Geometry check sheet. Reference: drawing and pictorial views, mm from the part's lowest x, y, z. A direction names the side the tool comes from. Round coordinates to 2 decimals unless told otherwise and drop trailing zeros. Write each loop counter-clockwise with the first axis right and the second up, starting at its lowest first coordinate (ties: lowest second). Pieces come first, ordered by that corner, then holes. Notation, with made-up numbers: (-38, 36) -> (8, 36) arc R24 ccw to (8, 59) -> close; hole circle Ø9 at (-2, 83.5). An arc over 180 degrees is marked (long way). Write item = value, one per line.
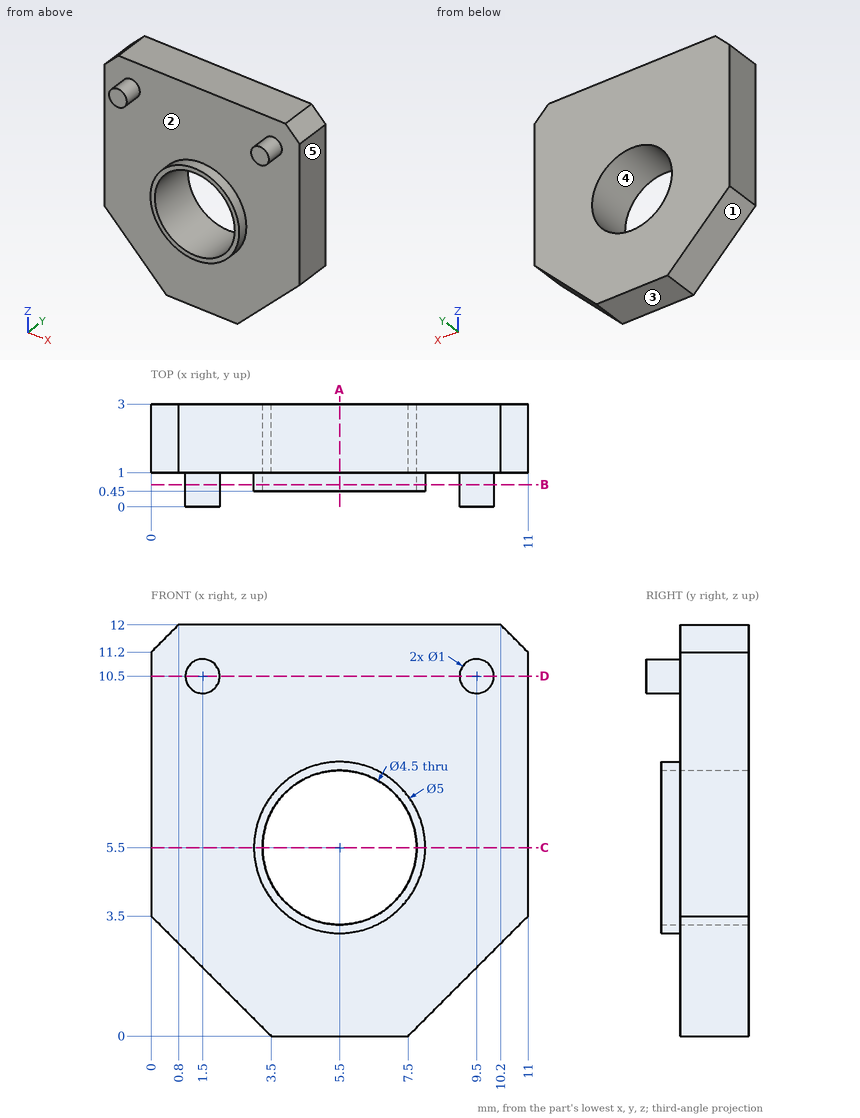
(1) Access from +Z, -Z, +X, -X, +Y, -Y to the whole of each face (thin tool, end or side, straight path). Record for the marked faces 1 and 2.
Worked answers:
face_1 = -Z, -X, +Y, -Y
face_2 = -Y
(2) Sectioned sample at A-A on x = 5.5. Enter the section's corners in (y, z), then the cut area to 3 significant figures.
Worked answers:
outline = (0.45, 3) -> (1, 3) -> (1, 0) -> (3, 0) -> (3, 3.25) -> (0.45, 3.25) -> close; (0.45, 7.75) -> (3, 7.75) -> (3, 12) -> (1, 12) -> (1, 8) -> (0.45, 8) -> close
area = 15.3 mm²
(3) Sectioned sample at D-D on z = 10.5. Enter the section's corners in (x, y).
Worked answers:
outline = (0, 1) -> (1, 1) -> (1, 0) -> (2, 0) -> (2, 1) -> (9, 1) -> (9, 0) -> (10, 0) -> (10, 1) -> (11, 1) -> (11, 3) -> (0, 3) -> close
(4) Material ranges on L1, parallel to Z at x = 5.5, y = 1.2; L2, parallel to X at y = 1.35, z = 5.5; L3, parallel to Z at x = 9.5, y = 2.55, recorded low to high. Write a range as [from, to].
Worked answers:
L1 = [0, 3.25], [7.75, 12]
L2 = [0, 3.25], [7.75, 11]
L3 = [2, 12]
(5) Release check for a two-part mould opening along X. For the marked faces 3, 4 and 5 record: pulls with the +X half, pulls with the -X half, needs draft (parallel to the pull), parting line crosses it, or undercut.
Worked answers:
face_3 = needs draft
face_4 = undercut
face_5 = pulls with the +X half
(6) Sectioned sample at B-B on y = 0.65. Enter the section's corners in (x, z), then the cut area to 3 significant figures.
Worked answers:
outline = circle Ø1 at (1.5, 10.5); circle Ø5 at (5.5, 5.5); circle Ø1 at (9.5, 10.5); hole circle Ø4.5 at (5.5, 5.5)
area = 5.30 mm²
(7) Sectioned sample at C-C on z = 5.5. Enter the section's corners in (x, y).
Worked answers:
outline = (0, 1) -> (3, 1) -> (3, 0.45) -> (3.25, 0.45) -> (3.25, 3) -> (0, 3) -> close; (7.75, 0.45) -> (8, 0.45) -> (8, 1) -> (11, 1) -> (11, 3) -> (7.75, 3) -> close
(8) Go/stop test with flat-tipped pins: P1, Ø5.5, axis at x = 6, z = 6.5, coming from the -Y side; P2, Ø1.5, axis at x = 5.5, y = 1, coming from the -Z side. Record where each tip stops, or that it passes through.
Worked answers:
P1 = 0.45
P2 = 0
